Part print with two shaded views. Sizes in mm from the minimum x, y, z corner. Give positions to 0.01 mm unless a question says otherwise; leave off trailing zeros. Loops run counter-clockwise (first coordinate to the right, second up) from the corner with the lowest first, then second, coordinate; pieces in that order, holes last. Notation, with made-up numbers: M 42,78.25 L 76,78.25 A13 ccw 76,91.25 Z; hole C 21.5,20.25 d2. An arc over 180 degrees is marked long. Answer in a Markdown table with one row per item.
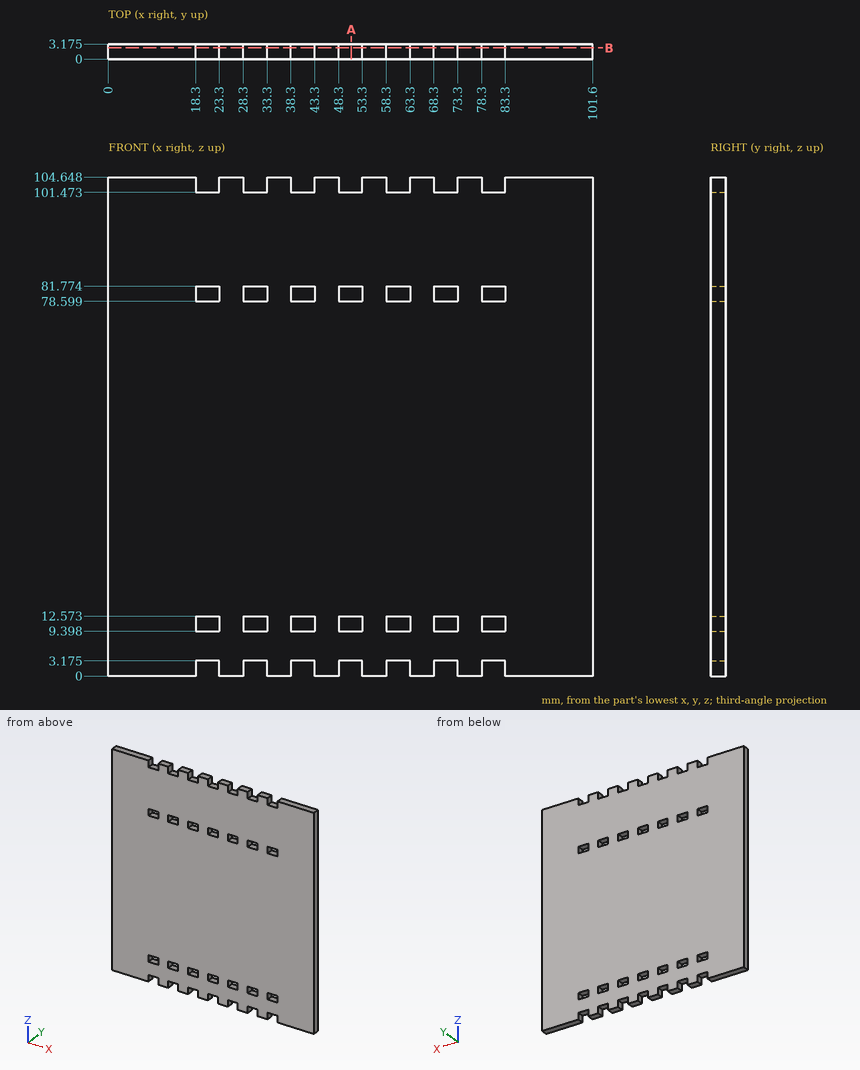
Q1. Probe probe 1 along Z at (x, y) = (69, 0.1) (3 decimals). List the from-to ranges inside material, lowest first.
Reported:
| item | result |
|---|---|
| probe 1 | 3.175 to 9.398, 12.573 to 78.599, 81.774 to 101.473 |
Q2. Saw through at B-B (y = 2.35). Give the number of separate pieces and of enclosed holes in the cut face, and give its area (3 significant figures).
Reported:
| item | result |
|---|---|
| separate pieces | 1 |
| enclosed holes | 14 |
| area | 10,200 mm² |
Q3. Drop flat-ended pins along their axis: pin 1 (1.6 mm diameter, centred on y = 1, z = 102.5, fed in from -X); pin 2 (1 mm diameter, centred on x = 50, y = 1, fed in from +Z); pin 3 (1.6 mm diameter, centred on x = 32, y = 1, fed in from -Z) (3 decimals). Give the stop position or say it passes through.
Reported:
| item | result |
|---|---|
| pin 1 | x = 0 |
| pin 2 | z = 101.47 |
| pin 3 | z = 3.175 |
Q4. Saw through at A-A (x = 51). Give the cut face in (y, z) (3 decimals), and give its area (3 significant figures).
Reported:
| item | result |
|---|---|
| outline | M 0,3.175 L 3.175,3.175 L 3.175,9.398 L 0,9.398 Z; M 0,12.573 L 3.175,12.573 L 3.175,78.599 L 0,78.599 Z; M 0,81.774 L 3.175,81.774 L 3.175,101.473 L 0,101.473 Z |
| area | 292 mm² |
